```python
from build123d import *

# Parameters (mm, degrees)
SKETCH1_W                 = 100
SKETCH1_H                 = 100
BOSS_EXTRUDE1_DEPTH       = 5
F_4_0MM_DOWEL_HOLE1_D     = 4
F_4_0MM_DOWEL_HOLE1_DEPTH = 5


with BuildPart() as part:
    # Sketch1 → Boss-Extrude1 (new body)
    with BuildSketch(Plane(origin=(0, 0, 0), x_dir=(1, 0, 0), z_dir=(0, 1, 0))):
        Rectangle(SKETCH1_W, SKETCH1_H)
    extrude(amount=BOSS_EXTRUDE1_DEPTH)

    # Ø4.0mm Dowel Hole1
    with Locations(Plane(origin=(-47.5, 5, -46), x_dir=(0, 0, 1), z_dir=(0, 1, 0))):
        with Locations((0, 0), (0, 95), (92, 95), (92, 0)):
            Hole(F_4_0MM_DOWEL_HOLE1_D / 2, depth=F_4_0MM_DOWEL_HOLE1_DEPTH)


solid = part.part
```
Geometry: final body of the model. Coordinates: model frame, mm. Round coordinates to 2 decimals unless told otherwise and drop trailing zeros. Order: outer loops, then holes, each group sorted by start corner. A loop starts at its lowest first (then second) coordinate and runs counter-clockwise, first axis right, second up. Notation, with made-up numbers: (-35, 37.25) -> (-6, 37.25) arc R8 cw to (-6, 43.25) -> close; hole circle Ø9 at (32, -24.5). An arc over 180 degrees is marked (long way). Use one line per item in the form item = value. Start each with the question number.
1. Cut plane B-B (z = -46). Return the cut outline in (x, y).
2. Line query: probe 1 along X at (y, z) = (1.95, -46). Output: solid intervals per line, ascending.
3. Draft query along X for faces 1 (the face through (50, 2, 1)), 2 (the face through (-49.452, 2.465, 46.434)), 3 (the face through (-1, 2, 50)). Return one class per face: pulls with the +X half, pulls with the -X half, needs draft (parallel to the pull), parting line crosses it, or undercut.
4. Pin query (flat end, axial travel): pin 1 Ø3 at (x, z) = (-47.5, 46) entering from -Y. Return the tip coordinate at first contact, or that it passes through.
5. Cut plane A-A (x = 47.5). Return the cut outline in (y, z).
Solution:
q1.outline = (-50, 0) -> (-49.5, 0) -> (-49.5, 5) -> (-50, 5) -> close; (-45.5, 0) -> (45.5, 0) -> (45.5, 5) -> (-45.5, 5) -> close; (49.5, 0) -> (50, 0) -> (50, 5) -> (49.5, 5) -> close
q2.probe_1 = -50 to -49.5, -45.5 to 45.5, 49.5 to 50
q3.face_1 = pulls with the +X half
q3.face_2 = undercut
q3.face_3 = needs draft
q4.pin_1 = through
q5.outline = (0, -50) -> (5, -50) -> (5, -48) -> (0, -48) -> close; (0, -44) -> (5, -44) -> (5, 44) -> (0, 44) -> close; (0, 48) -> (5, 48) -> (5, 50) -> (0, 50) -> close
